```python
from build123d import *

# Parameters (mm, degrees)
F0_R     = 3.175
F1_DEPTH = 16.51
F2_DEPTH = 2.54


# Not quite as in the source:
# - a feature names something its author has since deleted; it is built from what else it names


with BuildPart() as f1:
    # F0 (on Front) → F1 (new body)
    with BuildSketch(Plane.XZ):
        with BuildLine():
            Line((15.24, 10.16), (0, 10.16))
            Line((0, 10.16), (-15.24, 10.16))
            Line((-15.24, 10.16), (-15.24, -23.0504914403))
            add(Edge.make_bspline(
                [(-15.24, -23.0504914403), (-12.4936951429, -23.050233708), (-10.2976989889, -24.6278435924), (-8.636, -27.1888607202)],
                knots=[0, 0, 0, 0, 8.4526904957, 8.4526904957, 8.4526904957, 8.4526904957], degree=3))
            Line((-8.636, -27.1888607202), (-8.636, -21.770928055))
            ThreePointArc((-8.636, -21.770928055), (-11.43, -16.51), (-8.636, -11.249071945))
            Line((-8.636, -11.249071945), (-8.636, -5.260928055))
            ThreePointArc((-8.636, -5.260928055), (-11.1516304709, 1.8595169871), (-5.08, 6.35))
            Line((-5.08, 6.35), (5.08, 6.35))
            ThreePointArc((5.08, 6.35), (9.5701280605, 4.4901280605), (11.43, 0))
            ThreePointArc((11.43, 0), (9.5701280605, -4.4901280605), (5.08, -6.35))
            Line((5.08, -6.35), (-5.08, -6.35))
            ThreePointArc((-5.08, -6.35), (-5.2705858603, -6.3471392792), (-5.461, -6.3385596944))
            Line((-5.461, -6.3385596944), (-5.461, -10.1714403056))
            ThreePointArc((-5.461, -10.1714403056), (-5.2705858603, -10.1628607208), (-5.08, -10.16))
            Line((-5.08, -10.16), (5.08, -10.16))
            ThreePointArc((5.08, -10.16), (9.5701280605, -12.0198719395), (11.43, -16.51))
            ThreePointArc((11.43, -16.51), (9.5701280605, -21.0001280605), (5.08, -22.86))
            Line((5.08, -22.86), (-5.08, -22.86))
            ThreePointArc((-5.08, -22.86), (-5.2705858603, -22.8571392792), (-5.461, -22.8485596944))
            Line((-5.461, -22.8485596944), (-5.461, -35.926681818))
            add(Edge.make_bspline(
                [(-5.461, -35.926681818), (-3.0177559473, -48.8656738837), (-6.4817336355, -66.9757324356), (-15.24, -67.5004914403)],
                knots=[15.9624587288, 15.9624587288, 15.9624587288, 15.9624587288, 44.45, 44.45, 44.45, 44.45], degree=3))
            Line((-15.24, -67.5004914403), (-15.24, -80.2004914403))
            Line((-15.24, -80.2004914403), (0, -80.2004914403))
            Line((0, -80.2004914403), (15.24, -80.2004914403))
            Line((15.24, -80.2004914403), (15.24, -67.5004914403))
            add(Edge.make_bspline(
                [(15.24, -23.0504914403), (0.7980597731, -23.0491361081), (1.5742035665, -66.6816935827), (15.24, -67.5004914403)],
                knots=[0, 0, 0, 0, 44.45, 44.45, 44.45, 44.45], degree=3))
            Line((15.24, -23.0504914403), (15.24, 10.16))
        make_face()
        with Locations((-8.89, -73.8504914403)):
            Circle(F0_R, mode=Mode.SUBTRACT)
        with Locations((8.89, -73.8504914403)):
            Circle(F0_R, mode=Mode.SUBTRACT)
    extrude(amount=F1_DEPTH)

    # F0 (on Front) → F2 (join)
    with BuildSketch(Plane.XZ):
        with BuildLine():
            ThreePointArc((-5.08, 6.35), (-11.1516304709, 1.8595169871), (-8.636, -5.260928055))
            ThreePointArc((-8.636, -5.260928055), (-7.1209102718, -6.0130845048), (-5.461, -6.3385596944))
            ThreePointArc((-5.461, -6.3385596944), (-5.2705858603, -6.3471392792), (-5.08, -6.35))
            ThreePointArc((-5.08, -6.35), (-2.2401936686, -5.6796126628), (0, -3.81))
            ThreePointArc((0, -3.81), (-1.27, 0), (0, 3.81))
            ThreePointArc((0, 3.81), (-2.2401936686, 5.6796126628), (-5.08, 6.35))
        make_face()
        with BuildLine():
            ThreePointArc((5.08, 6.35), (2.2401936686, 5.6796126628), (0, 3.81))
            ThreePointArc((0, 3.81), (0.9441389426, 2.0080463142), (1.27, 0))
            ThreePointArc((1.27, 0), (0.9441389426, -2.0080463142), (0, -3.81))
            ThreePointArc((0, -3.81), (2.2401936686, -5.6796126628), (5.08, -6.35))
            ThreePointArc((5.08, -6.35), (9.5701280605, -4.4901280605), (11.43, 0))
            ThreePointArc((11.43, 0), (9.5701280605, 4.4901280605), (5.08, 6.35))
        make_face()
        with BuildLine():
            Line((5.08, 6.35), (-5.08, 6.35))
            ThreePointArc((-5.08, 6.35), (-2.2401936686, 5.6796126628), (0, 3.81))
            ThreePointArc((0, 3.81), (2.2401936686, 5.6796126628), (5.08, 6.35))
        make_face()
        with BuildLine():
            ThreePointArc((1.27, 0), (0.9441389426, 2.0080463142), (0, 3.81))
            ThreePointArc((0, 3.81), (-1.27, 0), (0, -3.81))
            ThreePointArc((0, -3.81), (0.9441389426, -2.0080463142), (1.27, 0))
        make_face()
        with BuildLine():
            ThreePointArc((0, -3.81), (-2.2401936686, -5.6796126628), (-5.08, -6.35))
            Line((-5.08, -6.35), (5.08, -6.35))
            ThreePointArc((5.08, -6.35), (2.2401936686, -5.6796126628), (0, -3.81))
        make_face()
        with BuildLine():
            Line((-5.461, -22.5981636269), (-5.461, -22.8485596944))
            ThreePointArc((-5.461, -22.8485596944), (-5.2705858603, -22.8571392792), (-5.08, -22.86))
            ThreePointArc((-5.08, -22.86), (-2.2401936686, -22.1896126628), (0, -20.32))
            ThreePointArc((0, -20.32), (-1.27, -16.51), (0, -12.7))
            ThreePointArc((0, -12.7), (-2.2401936686, -10.8303873372), (-5.08, -10.16))
            ThreePointArc((-5.08, -10.16), (-5.2705858603, -10.1628607208), (-5.461, -10.1714403056))
            Line((-5.461, -10.1714403056), (-5.461, -22.5981636269))
        make_face()
        with BuildLine():
            ThreePointArc((0, -12.7), (-1.27, -16.51), (0, -20.32))
            ThreePointArc((0, -20.32), (0.9441389426, -18.5180463142), (1.27, -16.51))
            ThreePointArc((1.27, -16.51), (0.9441389426, -14.5019536858), (0, -12.7))
        make_face()
        with BuildLine():
            Line((5.08, -10.16), (-5.08, -10.16))
            ThreePointArc((-5.08, -10.16), (-2.2401936686, -10.8303873372), (0, -12.7))
            ThreePointArc((0, -12.7), (2.2401936686, -10.8303873372), (5.08, -10.16))
        make_face()
        with BuildLine():
            ThreePointArc((1.27, -16.51), (0.9441389426, -18.5180463142), (0, -20.32))
            ThreePointArc((0, -20.32), (2.2401936686, -22.1896126628), (5.08, -22.86))
            ThreePointArc((5.08, -22.86), (9.5701280605, -21.0001280605), (11.43, -16.51))
            ThreePointArc((11.43, -16.51), (9.5701280605, -12.0198719395), (5.08, -10.16))
            ThreePointArc((5.08, -10.16), (2.2401936686, -10.8303873372), (0, -12.7))
            ThreePointArc((0, -12.7), (0.9441389426, -14.5019536858), (1.27, -16.51))
        make_face()
        with BuildLine():
            ThreePointArc((0, -20.32), (-2.2401936686, -22.1896126628), (-5.08, -22.86))
            Line((-5.08, -22.86), (5.08, -22.86))
            ThreePointArc((5.08, -22.86), (2.2401936686, -22.1896126628), (0, -20.32))
        make_face()
        with BuildLine():
            Line((-8.636, -21.770928055), (-8.636, -27.1888607202))
            add(Edge.make_bspline(
                [(-8.636, -27.1888607202), (-7.1596683768, -29.4641889225), (-6.1050779286, -32.5157580511), (-5.461, -35.926681818)],
                knots=[8.4526904957, 8.4526904957, 8.4526904957, 8.4526904957, 15.9624587288, 15.9624587288, 15.9624587288, 15.9624587288], degree=3))
            Line((-5.461, -35.926681818), (-5.461, -22.8485596944))
            ThreePointArc((-5.461, -22.8485596944), (-7.1209102718, -22.5230845048), (-8.636, -21.770928055))
        make_face()
        with BuildLine():
            Line((-8.636, -5.260928055), (-8.636, -11.249071945))
            ThreePointArc((-8.636, -11.249071945), (-7.1209102718, -10.4969154952), (-5.461, -10.1714403056))
            Line((-5.461, -10.1714403056), (-5.461, -6.3385596944))
            ThreePointArc((-5.461, -6.3385596944), (-7.1209102718, -6.0130845048), (-8.636, -5.260928055))
        make_face()
        with BuildLine():
            ThreePointArc((-8.636, -11.249071945), (-11.43, -16.51), (-8.636, -21.770928055))
            ThreePointArc((-8.636, -21.770928055), (-7.1209102718, -22.5230845048), (-5.461, -22.8485596944))
            Line((-5.461, -22.8485596944), (-5.461, -22.5981636269))
            Line((-5.461, -22.5981636269), (-5.461, -10.1714403056))
            ThreePointArc((-5.461, -10.1714403056), (-7.1209102718, -10.4969154952), (-8.636, -11.249071945))
        make_face()
    extrude(amount=F2_DEPTH)


solid = f1.part
```
Can you work these out from the model? Positions are in its coordinate system, mm. A direction names the side the tool comes from. Round coordinates to 2 decimals unless told otherwise and drop trailing zeros. Order: outer loops, then holes, each group sorted by start corner. A loop starts at its lowest first (then second) coordinate and runs counter-clockwise, first axis right, second up. Notation, with made-up numbers: (72.25, 60.25) -> (109.25, 60.25) arc R36 cw to (109.25, 94.25) -> close; hole circle Ø11 at (85.25, 26.25). An arc over 180 degrees is marked (long way). Return JSON: item names as keys, results as strings. Group by question number.
1. Will this pin go through, and if not, where does the flat tip stop? pin 1 (5 mm diameter, centred on x = -11.5, z = -32.5, fed in from +Y).
2. If we section it at A-A, the plane z = -72: Write out the boundary of the cut face in (x, y).
3. I need wall thicknesses on line 1 (Z direction, x = 0, y = -7); line 2 (X direction, y = -8, z = -9); line 3 (Z direction, x = -8.89, y = -13). Which ranges of each line are inside material? Lowest first, please. Write a range as [from, to].
4. We'd pull the mould along X, two halves only. Please class faces 1 (the face through (15.24, -8, -7)), 2 (the face through (0, -8, -80.2)), 3 (the face through (0, -9, -22.86)): released by +X, released by -X, zero draft, split by the parting line, or undercut.
5. If we section it at C-C, the plane x = 7: Count the separate pieces of the cut face and the enclosed holes in it, then the cut area to 3 significant figures.
6. If we section it at B-B, the plane x = 0.5: Write out the boundary of the cut face in (y, z).
7. Which directions (+Z, -Z, +X, -X, +Y, -Y) give clear straight access to the entire face, cutting with the end or side of a thin tool? Please do faces 4 (the face through (0, -9, 6.35)), 5 (the face through (0, 0, -24)).
Output values:
{
 "1": {"pin 1": "through"},
 "2": {"outline": "(-15.24, -16.51) -> (-11.47, -16.51) -> (-11.47, 0) -> (-15.24, 0) -> close; (-6.31, -16.51) -> (6.31, -16.51) -> (6.31, 0) -> (-6.31, 0) -> close; (11.47, -16.51) -> (15.24, -16.51) -> (15.24, 0) -> (11.47, 0) -> close"},
 "3": {"line 1": "[-80.2, -22.86], [-10.16, -6.35], [6.35, 10.16]", "line 2": "[-15.24, -8.64], [-5.46, 15.24]", "line 3": "[-80.2, -77.03], [-70.68, -63.03], [-26.81, -21.59], [-11.43, -5.08], [5.08, 10.16]"},
 "4": {"face 1": "released by +X", "face 2": "zero draft", "face 3": "undercut"},
 "5": {"separate pieces": "3", "enclosed holes": "0", "area": "596 mm²"},
 "6": {"outline": "(-16.51, -80.2) -> (0, -80.2) -> (0, 10.16) -> (-16.51, 10.16) -> (-16.51, 6.35) -> (-2.54, 6.35) -> (-2.54, -6.35) -> (-16.51, -6.35) -> (-16.51, -10.16) -> (-2.54, -10.16) -> (-2.54, -22.86) -> (-16.51, -22.86) -> close"},
 "7": {"face 4": "-Y", "face 5": "+Z, -Z, +X, -X, +Y"}
}
